from build123d import *

# Parameters (mm, degrees)
SKETCH1_W               = 193
SKETCH1_H               = 117.5
BOSS_EXTRUDE1_DEPTH     = 3.22
SKETCH3_W               = 193
SKETCH3_H               = 117.5
SKETCH3_W_2             = 187.6
SKETCH3_H_2             = 112.1
BOSS_EXTRUDE2_DEPTH     = 55
SKETCH4_R               = 3
SKETCH4_R_2             = 1.1
BOSS_EXTRUDE3_DEPTH     = 6.36
SKETCH6_R               = 4
SKETCH6_R_2             = 1
BOSS_EXTRUDE4_DEPTH     = 51.84
SKETCH7_R               = 4.7625
CUT_EXTRUDE1_DEPTH      = 56
CUT_EXTRUDE1_DEPTH_BACK = 4.22
F_1_4_CLEARANCE_HOLE1_D = 6.7564


with BuildPart() as part:
    # Sketch1 → Boss-Extrude1 (new body)
    with BuildSketch(Plane(origin=(0, 0, 0), x_dir=(1, 0, 0), z_dir=(0, 1, 0))):
        with Locations((96.5, 58.75)):
            Rectangle(SKETCH1_W, SKETCH1_H)
    extrude(amount=BOSS_EXTRUDE1_DEPTH)

    # Sketch3 → Boss-Extrude2 (add)
    with BuildSketch(Plane(origin=(0, 3.22, 0), x_dir=(1, 0, 0), z_dir=(0, 1, 0))):
        with Locations((96.5, 58.75)):
            Rectangle(SKETCH3_W, SKETCH3_H)
        with Locations((96.5, 58.75)):
            Rectangle(SKETCH3_W_2, SKETCH3_H_2, mode=Mode.SUBTRACT)
    extrude(amount=BOSS_EXTRUDE2_DEPTH)

    # Sketch4 → Boss-Extrude3 (add)
    with BuildSketch(Plane(origin=(0, 3.22, 0), x_dir=(1, 0, 0), z_dir=(0, 1, 0))):
        with Locations(Location((17.2, 17.7, 0), (0, 0, 90))):  # turned: the seam where the file's is
            Circle(SKETCH4_R)
        with Locations(Location((17.2, 17.7, 0), (0, 0, 270))):  # turned: the seam where the file's is
            Circle(SKETCH4_R_2, mode=Mode.SUBTRACT)
        with Locations(Location((175.8, 17.7, 0), (0, 0, 90))):  # turned: the seam where the file's is
            Circle(SKETCH4_R)
        with Locations(Location((175.8, 17.7, 0), (0, 0, 90))):  # turned: the seam where the file's is
            Circle(SKETCH4_R_2, mode=Mode.SUBTRACT)
        with Locations(Location((17.2, 99.8, 0), (0, 0, 90))):  # turned: the seam where the file's is
            Circle(SKETCH4_R)
        with Locations(Location((17.2, 99.8, 0), (0, 0, 90))):  # turned: the seam where the file's is
            Circle(SKETCH4_R_2, mode=Mode.SUBTRACT)
        with Locations(Location((175.8, 99.8, 0), (0, 0, 90))):  # turned: the seam where the file's is
            Circle(SKETCH4_R)
        with Locations(Location((175.8, 99.8, 0), (0, 0, 270))):  # turned: the seam where the file's is
            Circle(SKETCH4_R_2, mode=Mode.SUBTRACT)
    extrude(amount=BOSS_EXTRUDE3_DEPTH)

    # Sketch6 → Boss-Extrude4 (add)
    with BuildSketch(Plane(origin=(0, 3.22, 0), x_dir=(1, 0, 0), z_dir=(0, 1, 0))):
        with Locations(Location((8.7, 8.7, 0), (0, 0, 90))):  # turned: the seam where the file's is
            Circle(SKETCH6_R)
        with Locations(Location((8.7, 8.7, 0), (0, 0, 90))):  # turned: the seam where the file's is
            Circle(SKETCH6_R_2, mode=Mode.SUBTRACT)
        with Locations(Location((184.3, 8.7, 0), (0, 0, 90))):  # turned: the seam where the file's is
            Circle(SKETCH6_R)
        with Locations(Location((184.3, 8.7, 0), (0, 0, 90))):  # turned: the seam where the file's is
            Circle(SKETCH6_R_2, mode=Mode.SUBTRACT)
        with Locations(Location((184.3, 108.8, 0), (0, 0, 90))):  # turned: the seam where the file's is
            Circle(SKETCH6_R)
        with Locations(Location((184.3, 108.8, 0), (0, 0, 90))):  # turned: the seam where the file's is
            Circle(SKETCH6_R_2, mode=Mode.SUBTRACT)
        with Locations(Location((8.7, 108.8, 0), (0, 0, 90))):  # turned: the seam where the file's is
            Circle(SKETCH6_R)
        with Locations(Location((8.7, 108.8, 0), (0, 0, 90))):  # turned: the seam where the file's is
            Circle(SKETCH6_R_2, mode=Mode.SUBTRACT)
    extrude(amount=BOSS_EXTRUDE4_DEPTH)

    # Sketch7 → Cut-Extrude1 (cut, two sides)
    with BuildSketch(Plane(origin=(0, 3.22, 0), x_dir=(1, 0, 0), z_dir=(0, 1, 0))) as cut_extrude1_sk:
        with Locations(Location((45, 45, 0), (0, 0, 270))):  # turned: the seam where the file's is
            Circle(SKETCH7_R)
    extrude(amount=CUT_EXTRUDE1_DEPTH, mode=Mode.SUBTRACT)
    extrude(cut_extrude1_sk.sketch, amount=-CUT_EXTRUDE1_DEPTH_BACK, mode=Mode.SUBTRACT)

    # 1/4 Clearance Hole1 (through all)
    with Locations(Plane(origin=(0, 3.22, 0), x_dir=(1, 0, 0), z_dir=(0, 1, 0))):
        with Locations((58.01, 45), (31.99, 45)):
            Hole(F_1_4_CLEARANCE_HOLE1_D / 2)


solid = part.part
Check sheet for the modelled part. Datum: model origin and axes. Units: mm. A direction names the side the tool comes from. Round coordinates to 2 decimals unless told otherwise and drop trailing zeros. Order: outer loops, then holes, each group sorted by start corner. A loop starts at its lowest first (then second) coordinate and runs counter-clockwise, first axis right, second up.
(1) Cross-section at B-B, the plane x = 45. Enter the section's corners in (y, z), and give its area (3 significant figures).
(2) Go/stop test with flat-tipped pins: P1, Ø0.7, axis at x = 176, z = -17.5, coming from the +Y side; P2, Ø2.5, axis at x = 185, z = -109.5, coming from the +Y side; P3, Ø6.5, axis at x = 175, z = -100.5, coming from the +Y side. Record where each tip stops, or that it passes through.
(3) Cross-section at C-C, the plane z = -30.5. Enter the section's corners in (x, y), and give its area (3 significant figures).
(4) Scan lines: probe 1 along Z at (x, y) = (39, 7.5); probe 2 along X at (y, z) = (5, -99.8); probe 3 along Z at (x, y) = (31.99, 1.45). Record each from-to range of solid material in increasing order.
(5) Cross-section at A-A, the plane y = 51.5. State how many separate pieces and enclosed holes the cut face has, and give its area (3 significant figures).
(6) Draft check along X on faces 1 (the cylindrical face through (188.205, 28.777, -7.833)), 2 (the flat face through (96, 58.22, -116)), 3 (the flat face through (0, 29, -58)). Enter one of: pulls with the +X half, pulls with the -X half, needs draft (parallel to the pull), parting line crosses it, or undercut.
(7) Access from +Z, -Z, +X, -X, +Y, -Y to the whole of each face (thin tool, end or side, straight path). Record for faces 4 (the flat face through (193, 29, -58)), 5 (the cylindrical face through (8.524, 28.777, -104.804)).
Check sheet entries:
1. outline: (0, -117.5) - (58.22, -117.5) - (58.22, -114.8) - (3.22, -114.8) - (3.22, -49.76) - (0, -49.76) - close; (0, -40.24) - (3.22, -40.24) - (3.22, -2.7) - (58.22, -2.7) - (58.22, 0) - (0, 0) - close
1. area: 645 mm2
2. P1: stops at y = 3.22
2. P2: stops at y = 55.06
2. P3: stops at y = 9.58
3. outline: (0, 0) - (193, 0) - (193, 58.22) - (190.3, 58.22) - (190.3, 3.22) - (2.7, 3.22) - (2.7, 58.22) - (0, 58.22) - close
3. area: 918 mm2
4. probe 1: z = -117.5 to -114.8, -2.7 to 0
4. probe 2: x = 0 to 2.7, 14.2 to 16.1, 18.3 to 20.2, 172.8 to 174.7, 176.9 to 178.8, 190.3 to 193
4. probe 3: z = -117.5 to -48.38, -41.62 to 0
5. separate pieces: 5
5. enclosed holes: 5
5. area: 1,840 mm2
6. face 1: undercut
6. face 2: needs draft
6. face 3: pulls with the -X half
7. face 4: +Z, -Z, +X, +Y, -Y
7. face 5: +Y
